Here's the drawing with two shaded views (mm, measured from the low corner). I have some questions. Coordinates: 2 decimals unless noted, no trailing zeros. Order: outer loops, then holes, each group sorted by start corner. A loop starts at its lowest first (then second) coordinate and runs counter-clockwise, first axis right, second up. Notation, with made-up numbers: (57, -5) -> (71, -5) arc R29 cw to (71, 21) -> close; hole circle Ø9 at (39.25, 50). An arc over 180 degrees is marked (long way). Answer as a JSON object with one key per item and string values. Group by question number.
(1) I need wall thicknesses on line 1 (X direction, y = 3.2, z = 3.5) (1 decimal); line 2 (X direction, y = 3.5, z = 50.8); line 3 (Z direction, x = 66, y = 3.3) (1 decimal). Which ranges of each line are inside material? Lowest first, please.
(2) For pin 1 (1.4 mm diameter, centred on x = 27, y = 2.5, fed in from +Z); pin 2 (1.4 mm diameter, centred on x = 28.5, y = 3, fed in from -Z), each with a flat end and sliding along its axis, tell me the tip position at first contact or that it passes through.
(3) I want a section at A-A, the plane z = 50.8. List the corners of the cut face in (x, y) for me.
(4) I want a section at B-B, the plane y = 3.85. List the corners of the cut face in (x, z) for me (1 decimal), plus the area to 3 significant figures.
(5) I want a section at C-C, the plane z = 11.43. List the corners of the cut face in (x, y) for me, plus the area to 3 significant figures.
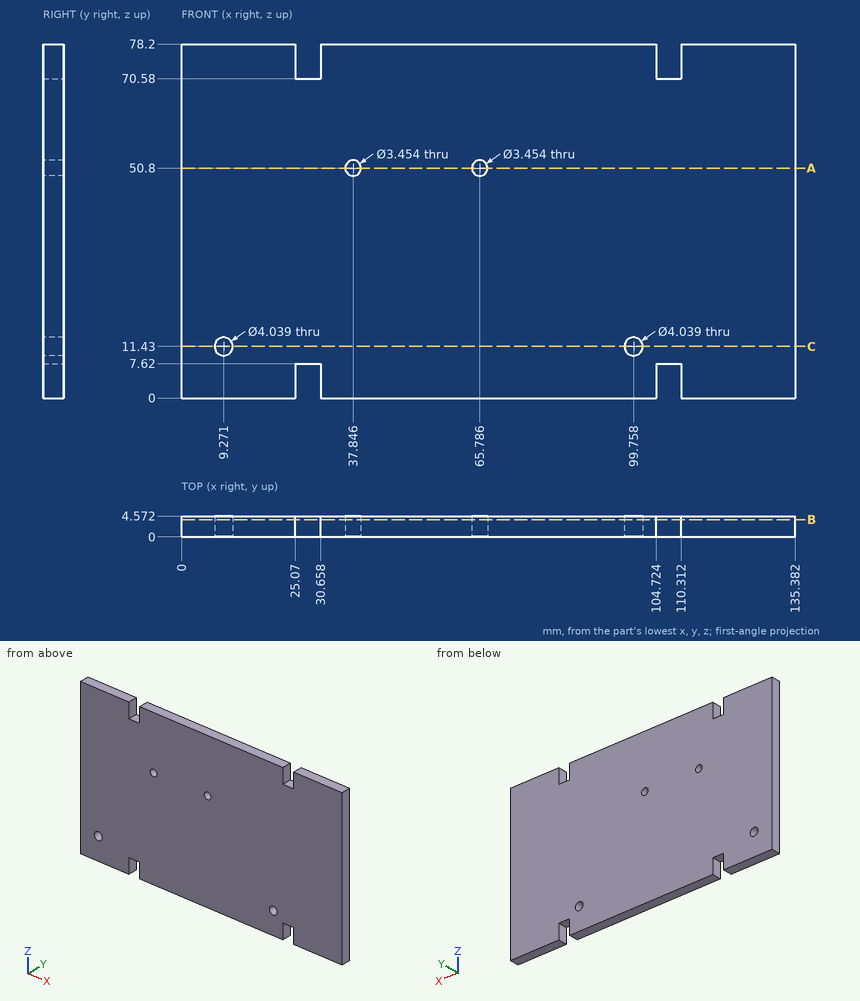
Computed values:
{
 "1": {"line 1": "x = 0 to 25.1, 30.7 to 104.7, 110.3 to 135.4", "line 2": "x = 0 to 36.12, 39.57 to 64.06, 67.51 to 135.38", "line 3": "z = 0 to 49.1, 52.5 to 78.2"},
 "2": {"pin 1": "stops at z = 70.58", "pin 2": "stops at z = 7.62"},
 "3": {"outline": "(0, 0) -> (36.12, 0) -> (36.12, 4.57) -> (0, 4.57) -> close; (39.57, 0) -> (64.06, 0) -> (64.06, 4.57) -> (39.57, 4.57) -> close; (67.51, 0) -> (135.38, 0) -> (135.38, 4.57) -> (67.51, 4.57) -> close"},
 "4": {"outline": "(0, 0) -> (25.1, 0) -> (25.1, 7.6) -> (30.7, 7.6) -> (30.7, 0) -> (104.7, 0) -> (104.7, 7.6) -> (110.3, 7.6) -> (110.3, 0) -> (135.4, 0) -> (135.4, 78.2) -> (110.3, 78.2) -> (110.3, 70.6) -> (104.7, 70.6) -> (104.7, 78.2) -> (30.7, 78.2) -> (30.7, 70.6) -> (25.1, 70.6) -> (25.1, 78.2) -> (0, 78.2) -> close; hole circle Ø4 at (9.3, 11.4); hole circle Ø3.5 at (37.8, 50.8); hole circle Ø3.5 at (65.8, 50.8); hole circle Ø4 at (99.8, 11.4)", "area": "10,400 mm2"},
 "5": {"outline": "(0, 0) -> (7.25, 0) -> (7.25, 4.57) -> (0, 4.57) -> close; (11.29, 0) -> (97.74, 0) -> (97.74, 4.57) -> (11.29, 4.57) -> close; (101.78, 0) -> (135.38, 0) -> (135.38, 4.57) -> (101.78, 4.57) -> close", "area": "582 mm2"}
}
